Input: part model. Units: mm. Frame: model coordinates. Face numbers are marked on the shaded views. A direction names the side the tool comes from. Give positions to 0.01 mm unless a question says otherwise; leave off trailing zeros. Loops run counter-clockwise (first coordinate to the right, second up) from the corner with the lowest first, then second, coordinate; pieces in that order, holes last. Notation, with made-up numbers: M 29,-18 L 84,-18 A30 cw 84,12 Z; hole C 38,-2.5 d10. An arc over 180 degrees is marked long. Answer as a JSON object with one key per item and string values. Group by question number.
1) First-contact query: P1, Ø3, axis at x = 16.5, z = -2, coming from the +Y side; P2, Ø3, axis at x = -14, z = 1, coming from the +Y side; P3, Ø10, axis at x = -5.5, y = 8.5, coming from the +Z side. Flat tips, straight axial feed; report the tip coordinate or a pass-through.
2) Ray query, L1, parallel to X at y = 0, z = 0.75; L2, parallel to X at y = 0, z = 3.55 (3 decimals); L3, parallel to X at y = 0, z = 3.5 (3 decimals). Return the intervals inside material, ascending.
3) Access query for the marked faces 1 and 2. Directions: +Z, -Z, +X, -X, +Y, -Y. A direction counts if a zero-diameter tool reaches every point of the face in a straight line with its end or side. Return the directions, or none.
4) Section query C-C on z = 1.75. Return loops of the section in (x, y), plus the area to 3 significant figures.
5) Draft query along Y for the marked faces 3 and 4. Return one class per face: +Y half, -Y half, draft (parallel to the pull), parting line (faces both ways), or undercut.
from build123d import *


with BuildPart() as part:
    # Sketch1 → Revolve1 (revolve)
    with BuildSketch(Plane(origin=(0, 0, 0), x_dir=(0, 0, -1), z_dir=(1, 0, 0))):
        with BuildLine():
            ThreePointArc((-3.640744937, 20.3), (-3.552876972, 20.087867966), (-3.340744937, 20))
            Line((-3.340744937, 20), (3.059255063, 20))
            ThreePointArc((3.059255063, 20), (3.271387097, 20.087867966), (3.359255063, 20.3))
            Line((3.359255063, 20.3), (3.359255063, 21.055000054))
            Line((3.359255063, 21.055000054), (3.159255063, 21.055000054))
            Line((3.159255063, 21.055000054), (3.159255063, 24.650000054))
            Line((3.159255063, 24.650000054), (3.359255063, 24.650000054))
            Line((3.359255063, 24.650000054), (3.359255063, 25.7))
            ThreePointArc((3.359255063, 25.7), (3.271387097, 25.912132034), (3.059255063, 26))
            Line((3.059255063, 26), (-3.340744937, 26))
            ThreePointArc((-3.340744937, 26), (-3.552876972, 25.912132034), (-3.640744937, 25.7))
            Line((-3.640744937, 25.7), (-3.640744937, 24.650000054))
            Line((-3.640744937, 24.650000054), (-3.440744937, 24.650000054))
            Line((-3.440744937, 24.650000054), (-3.440744937, 21.055000054))
            Line((-3.440744937, 21.055000054), (-3.640744937, 21.055000054))
            Line((-3.640744937, 21.055000054), (-3.640744937, 20.3))
        make_face()
    revolve(axis=Axis((0, 0, 0), (0, 0, -1)))


solid = part.part
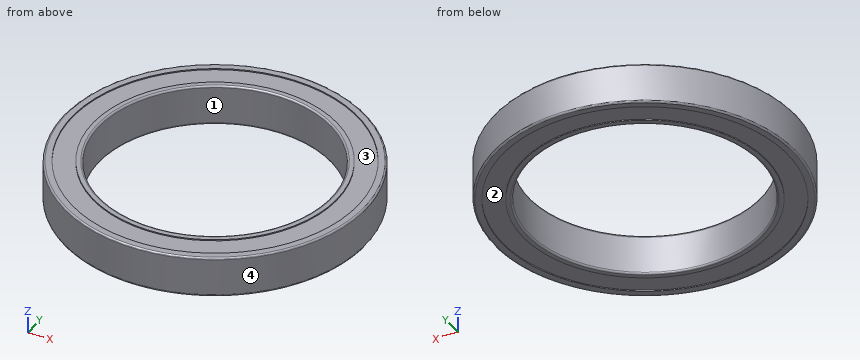
Output:
{
 "1": {"P1": "stops at y = 21.24", "P2": "stops at y = 22.8", "P3": "passes through"},
 "2": {"L1": "x = -26 to -20, 20 to 26", "L2": "x = -25.915 to -24.65, -21.055 to -20.085, 20.085 to 21.055, 24.65 to 25.915", "L3": "x = -25.954 to -24.65, -21.055 to -20.046, 20.046 to 21.055, 24.65 to 25.954"},
 "3": {"face 1": "+Z, -Z", "face 2": "-Z"},
 "4": {"outline": "C 0,0 d52; hole C 0,0 d40", "area": "867 mm^2"},
 "5": {"face 3": "undercut", "face 4": "parting line"}
}
